```python
from build123d import *

# Parameters (mm, degrees)
F0_W     = 50
F0_H     = 7.5
F1_DEPTH = 7
F2_W     = 38
F2_H     = 3
F3_DEPTH = 24
F5_DEPTH = 25
F6_R     = 2
F7_DEPTH = 3
F8_W     = 10
F8_H     = 7.5
F9_DEPTH = 9.9


with BuildPart() as f1:
    # F0 (on Top) → F1 (new body)
    with BuildSketch(Plane.XY):
        Rectangle(F0_W, F0_H)
    extrude(amount=F1_DEPTH)

    # F2 (on face) → F3 (join)
    with BuildSketch(Plane(origin=(0, 0, 0), x_dir=(1, 0, 0), z_dir=(0, 0, -1))):
        with Locations((-4, 0)):
            Rectangle(F2_W, F2_H)
    extrude(amount=F3_DEPTH)

    # F4 (on face) → F5 (cut)
    with BuildSketch(Plane.XZ.offset(1.5)):
        with BuildLine():
            add(Edge.make_bspline(
                [(-23, 0), (-21.1907899678, -16.0032901913), (-19.0204773098, -22.5683785975), (0, -24)],
                knots=[0, 0, 0, 0, 33.2415402772, 33.2415402772, 33.2415402772, 33.2415402772], degree=3))
            Line((-23, 0), (-23, -24))
            Line((-23, -24), (0, -24))
        make_face()
        with BuildLine():
            Line((15, 0), (2.7631570119, 0))
            add(Edge.make_bspline(
                [(7.8289462253, -24), (-4.1600125842, -18.4321980923), (-3.5605092999, -5.8886152692), (2.7631570119, 0)],
                knots=[0, 0, 0, 0, 24.5288038916, 24.5288038916, 24.5288038916, 24.5288038916], degree=3))
            Line((7.8289462253, -24), (15, -24))
            Line((15, -24), (15, 0))
        make_face()
    extrude(amount=-F5_DEPTH, mode=Mode.SUBTRACT)

    # F6 (on face) → F7 (cut)
    with BuildSketch(Plane(origin=(-25, 0, 0), x_dir=(0, -1, 0), z_dir=(-1, 0, 0))):
        with Locations((0, 3.5)):
            Circle(F6_R)
    extrude(amount=-F7_DEPTH, mode=Mode.SUBTRACT)

    # F8 (on face) → F9 (join)
    with BuildSketch(Plane.XY.offset(7)):
        with Locations((-20, 0)):
            Rectangle(F8_W, F8_H)
    extrude(amount=F9_DEPTH)


solid = f1.part
```
The listing builds one solid part. Answer for the finished solid, in the listing's coordinates (mm). A direction names the side the tool comes from. Coordinates: 2 decimals unless noted, no trailing zeros. Loops run counter-clockwise (first coordinate to the right, second up) from the corner with the lowest first, then second, coordinate; pieces in that order, holes last. Notation, with made-up numbers: (35.5, 16) -> (71.5, 16) arc R26 cw to (71.5, 46) -> close; hole circle Ø7 at (10, 62). An arc over 180 degrees is marked (long way). Return JSON: item names as keys, results as strings. Group by question number.
(1) Find the intervals of material crossed by probe 1 along Z at (x, y) = (-8, -1.75); probe 2 along Y at (x, z) = (-23, 3); probe 3 along Z at (x, y) = (4, -0.75), in increasing order. Write a range as from..to.
(2) Given pin 1 Ø3 at (y, z) = (-1.5, -10) entering from -X; pin 2 Ø4 at (x, y) = (6.5, 0) entering from +Z; pin 3 Ø1 at (y, z) = (0.5, -12) entering from -X, each flat-ended and moving along its own axis, determine where each tip first touches the part or whether it passes through.
(3) A cutting plane is placed at B-B on x = 13. Write down the section's boundary in (y, z).
(4) Which of the six approach directions +Z, -Z, +X, -X, +Y, -Y give full straight-line access (tool end or side, diameter ignored) to faces 1 (the flat face through (-11, 1.5, -12)), 2 (the flat face through (-11, -1.5, -12)), 3 (the cylindrical face through (-23.521, -1.908, 4.101)), 4 (the flat face through (-15, 0, 12))?
(5) A cutting plane is placed at A-A on z = 3.5. Write down the section's boundary in (x, y), and give its area (3 significant figures).
(6) Determine the mould class of faces 5 (the flat face through (-6, 3.75, 5)), 6 (the flat face through (4, 0, -24)), 7 (the flat face through (5, 0, 7)), 8 (the flat face through (-22, 0, 4)) for opening direction Z: released by +Z, released by -Z, zero draft, split by the parting line, or undercut.
(7) A cutting plane is placed at C-C on z = 13.5. Write down the section's boundary in (x, y), and give its area (3 significant figures).
The answers:
{
 "1": {"probe 1": "z = 0..7", "probe 2": "y = -3.75..-1.94, 1.94..3.75", "probe 3": "z = -24..-21.68, 0..7"},
 "2": {"pin 1": "stops at x = -21.74", "pin 2": "stops at z = 7", "pin 3": "stops at x = -20.98"},
 "3": {"outline": "(-3.75, 0) -> (3.75, 0) -> (3.75, 7) -> (-3.75, 7) -> close"},
 "4": {"face 1": "-Z, +X, -X, +Y", "face 2": "-Z, +X, -X, -Y", "face 3": "-X", "face 4": "+Z, +X, +Y, -Y"},
 "5": {"outline": "(-25, -3.75) -> (25, -3.75) -> (25, 3.75) -> (-25, 3.75) -> (-25, 2) -> (-22, 2) -> (-22, -2) -> (-25, -2) -> close", "area": "363 mm^2"},
 "6": {"face 5": "zero draft", "face 6": "released by -Z", "face 7": "released by +Z", "face 8": "undercut"},
 "7": {"outline": "(-25, -3.75) -> (-15, -3.75) -> (-15, 3.75) -> (-25, 3.75) -> close", "area": "75.0 mm^2"}
}
